Can you work these out from the model? Positions are in its coordinate system, mm. Coordinates: 2 decimals unless noted, no trailing zeros. Order: outer loops, then holes, each group sorted by start corner. A loop starts at its lowest first (then second) coordinate and runs counter-clockwise, first axis right, second up. Notation, with made-up numbers: M -4,-9.75 L 16,-9.75 A22 cw 16,6.25 Z; hole C 86,76.5 d8. An arc over 180 degrees is marked long. Answer as a JSON object with one key per item and string values.
from build123d import *

# Parameters (mm, degrees)
SKETCH1_R           = 2.5
BOSS_EXTRUDE1_DEPTH = 3.175
FILLET1_R           = 10
SKETCH2_W           = 9
SKETCH2_H           = 21
CUT_EXTRUDE1_DEPTH  = 90.108082017
FILLET2_R           = 10
SKETCH4_W           = 90.343709808
SKETCH4_H           = 29.159436912
CUT_EXTRUDE3_DEPTH  = 83
CUT_EXTRUDE4_DEPTH  = 90.108082017


with BuildPart() as part:
    # Sketch1 → Boss-Extrude1 (new body)
    with BuildSketch(Plane.XY):
        with BuildLine():
            Line((-9.56, -38.262636689), (-9.56, -41.437636689))
            Line((-9.56, -41.437636689), (9.56, -41.437636689))
            Line((9.56, -41.437636689), (9.56, -38.262636689))
            Line((9.56, -38.262636689), (12.735, -38.262636689))
            Line((12.735, -38.262636689), (12.735, -41.437636689))
            Line((12.735, -41.437636689), (15.91, -41.437636689))
            Line((15.91, -41.437636689), (21.91, -41.437636689))
            Line((21.91, -41.437636689), (21.91, -32.437636689))
            Line((21.91, -32.437636689), (18.735, -32.437636689))
            Line((18.735, -32.437636689), (18.735, -20.437636689))
            Line((18.735, -20.437636689), (21.91, -20.437636689))
            Line((21.91, -20.437636689), (21.91, -9.437636689))
            Line((21.91, -9.437636689), (40, -9.437636689))
            Line((40, -9.437636689), (40, 30.562363311))
            Line((40, 30.562363311), (10, 30.562363311))
            Line((10, 30.562363311), (10, 45.562363311))
            Line((10, 45.562363311), (10, 48.89577614))
            Line((10, 48.89577614), (22.410269523, 48.89577614))
            ThreePointArc((22.410269523, 48.89577614), (26.000000001, 52.562363311), (22.410269523, 56.228950483))
            Line((22.410269523, 56.228950483), (11.727794547, 56.228950483))
            Line((11.727794547, 56.228950483), (11.727794547, 59.562363311))
            Line((11.727794547, 59.562363311), (10, 59.562363311))
            Line((10, 59.562363311), (8.552794547, 59.562363311))
            Line((8.552794547, 59.562363311), (8.552794547, 62.737363311))
            Line((8.552794547, 62.737363311), (11.727794547, 62.737363311))
            Line((11.727794547, 62.737363311), (11.727794547, 74.562363311))
            Line((11.727794547, 74.562363311), (40, 74.562363311))
            Line((40, 74.562363311), (40, 79.562363311))
            Line((40, 79.562363311), (0, 79.562363311))
            Line((0, 79.562363311), (-40, 79.562363311))
            Line((-40, 79.562363311), (-40, 74.562363311))
            Line((-40, 74.562363311), (-11.727794547, 74.562363311))
            Line((-11.727794547, 74.562363311), (-11.727794547, 62.737363311))
            Line((-11.727794547, 62.737363311), (-8.552794547, 62.737363311))
            Line((-8.552794547, 62.737363311), (-8.552794547, 59.562363311))
            Line((-8.552794547, 59.562363311), (-10, 59.562363311))
            Line((-10, 59.562363311), (-11.727794547, 59.562363311))
            Line((-11.727794547, 59.562363311), (-11.727794547, 56.228950483))
            Line((-11.727794547, 56.228950483), (-22.410269523, 56.228950483))
            ThreePointArc((-22.410269523, 56.228950483), (-26.000000001, 52.562363311), (-22.410269523, 48.89577614))
            Line((-22.410269523, 48.89577614), (-10, 48.89577614))
            Line((-10, 48.89577614), (-10, 45.562363311))
            Line((-10, 45.562363311), (-10, 30.562363311))
            Line((-10, 30.562363311), (-40, 30.562363311))
            Line((-40, 30.562363311), (-40, -9.437636689))
            Line((-40, -9.437636689), (-21.91, -9.437636689))
            Line((-21.91, -9.437636689), (-21.91, -20.437636689))
            Line((-21.91, -20.437636689), (-18.735, -20.437636689))
            Line((-18.735, -20.437636689), (-18.735, -32.437636689))
            Line((-18.735, -32.437636689), (-21.91, -32.437636689))
            Line((-21.91, -32.437636689), (-21.91, -41.437636689))
            Line((-21.91, -41.437636689), (-15.91, -41.437636689))
            Line((-15.91, -41.437636689), (-12.735, -41.437636689))
            Line((-12.735, -41.437636689), (-12.735, -38.262636689))
            Line((-12.735, -38.262636689), (-9.56, -38.262636689))
        make_face()
        with BuildLine():
            Line((4, 1.562363311), (-4, 1.562363311))
            ThreePointArc((-4, 1.562363311), (-4.707106781, 1.85525653), (-5, 2.562363311))
            Line((-5, 2.562363311), (-5, 3.562363311))
            ThreePointArc((-5, 3.562363311), (-4.707106781, 4.269470092), (-4, 4.562363311))
            Line((-4, 4.562363311), (4, 4.562363311))
            ThreePointArc((4, 4.562363311), (4.707106781, 4.269470092), (5, 3.562363311))
            Line((5, 3.562363311), (5, 2.562363311))
            ThreePointArc((5, 2.562363311), (4.707106781, 1.85525653), (4, 1.562363311))
        make_face(mode=Mode.SUBTRACT)
        with Locations((-22, 52.562363311)):
            Circle(SKETCH1_R, mode=Mode.SUBTRACT)
        with Locations((22, 52.562363311)):
            Circle(SKETCH1_R, mode=Mode.SUBTRACT)
    extrude(amount=BOSS_EXTRUDE1_DEPTH)

    # Fillet1
    # the kernel refuses this fillet: 10 mm, written as the material it takes off along each edge
    with BuildSketch(Plane(origin=(-40, 79.562363311, -21.650635095), x_dir=(0, -1, 0), z_dir=(0, 0, 1))) as fillet1_piece_1:
        with BuildLine():
            CenterArc((10, 8.660254038), FILLET1_R, 180, 60)
            Line((0, 8.660254038), (-0.2, 8.660254038))
            Line((-0.2, 8.660254038), (-0.2, 0))
            Line((-0.2, 0), (0, -0.2))
            ThreePointArc((0, -0.2), (2.5, -0.2), (4.9, -0.173205081))
            Line((4.9, -0.173205081), (5, 0))
        make_face()
    extrude(amount=46.476270189, mode=Mode.SUBTRACT)
    with BuildSketch(Plane(origin=(40, 79.562363311, -21.650635095), x_dir=(-1, 0, 0), z_dir=(0, 0, 1))) as fillet1_piece_2:
        with BuildLine():
            CenterArc((8.660254038, 10), FILLET1_R, 210, 60)
            Line((0, 5), (-0.173205081, 4.9))
            ThreePointArc((-0.173205081, 4.9), (-0.2, 2.5), (-0.2, 0))
            Line((-0.2, 0), (0, -0.2))
            Line((0, -0.2), (8.660254038, -0.2))
            Line((8.660254038, -0.2), (8.660254038, 0))
        make_face()
    extrude(amount=46.476270189, mode=Mode.SUBTRACT)

    # Sketch2 → Cut-Extrude1 (cut, through all)
    with BuildSketch(Plane.XY.offset(3.175)):
        with Locations((-12.61, -26.137636689)):
            Rectangle(SKETCH2_W, SKETCH2_H)
    extrude(amount=-CUT_EXTRUDE1_DEPTH, mode=Mode.SUBTRACT)

    # Fillet2
    fillet2_edges = [part.edges().sort_by_distance(p)[0] for p in [
        (40, 30.562363311, 1.5875),
        (40, -9.437636689, 1.5875),
        (-40, -9.437636689, 1.5875),
        (-40, 30.562363311, 1.5875),
    ]]
    fillet(fillet2_edges, radius=FILLET2_R)

    # Sketch4 → Cut-Extrude3 (cut)
    with BuildSketch(Plane.XZ.offset(41.437636689)):
        Rectangle(SKETCH4_W, SKETCH4_H)
    extrude(amount=-CUT_EXTRUDE3_DEPTH, mode=Mode.SUBTRACT)

    # Sketch5 → Cut-Extrude4 (cut, through all)
    with BuildSketch(Plane.XY.offset(3.175)):
        Polygon((6.2, 68.212363311), (-6.2, 68.212363311), (-6.2, 45.562363311), (-3, 45.562363311), (-3, 40.562363311), (-0.113822398, 40.562363311), (0.113822398, 40.562363311), (3, 40.562363311), (3, 45.562363311), (6.2, 45.562363311), align=None)
    extrude(amount=-CUT_EXTRUDE4_DEPTH, mode=Mode.SUBTRACT)


solid = part.part
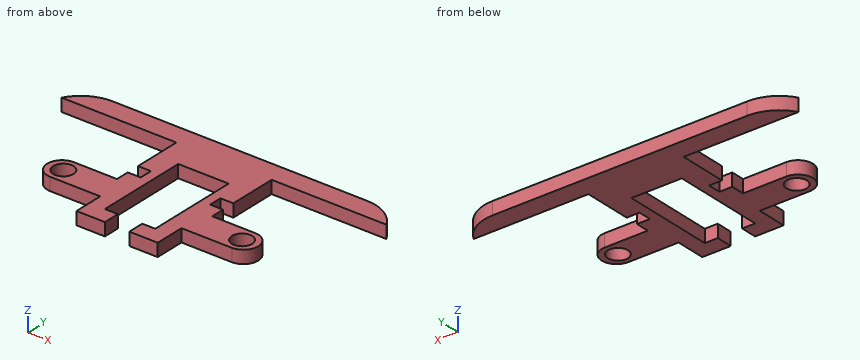
Item 1: I'm going to push flat-ended pins straight in: pin 1 (1 mm diameter, centred on y = 74, z = 0.5, fed in from -X); pin 2 (1 mm diameter, centred on y = 61, z = 1, fed in from -X); pin 3 (1.6 mm diameter, centred on y = 61, z = 1.5, fed in from +X). Where does each tip first touch, or does it pass through?
Answers follow:
{"pin 1": "stops at x = -11.73", "pin 2": "stops at x = -8.55", "pin 3": "stops at x = 8.55"}
Item 2: I want a section at C-C, the plane z = 1.9. Give the number of separate pieces and of enclosed holes in the cut face, plus the area to 3 significant figures.
Answers follow:
{"separate pieces": "1", "enclosed holes": "2", "area": "957 mm^2"}
Item 3: I want a section at B-B, the plane y = 67. Write out the boundary of the cut face in (x, z) (3 decimals).
Answers follow:
{"outline": "M -11.728,0 L -6.2,0 L -6.2,3.175 L -11.728,3.175 Z; M 6.2,0 L 11.728,0 L 11.728,3.175 L 6.2,3.175 Z"}
Item 4: I want a section at A-A, the plane y = 48. Write out the boundary of the cut face in (x, z) (3 decimals).
Answers follow:
{"outline": "M -10,0 L -6.2,0 L -6.2,3.175 L -10,3.175 Z; M 6.2,0 L 10,0 L 10,3.175 L 6.2,3.175 Z"}
Item 5: Please list where these lines run through material, in increasing order: line 1 (Y direction, x = 22, z = 2.15); line 2 (X direction, y = 58.5, z = 1.45); line 3 (Y direction, x = 16, z = 2.25).
Answers follow:
{"line 1": "y = 48.9 to 50.06, 55.06 to 56.23, 74.56 to 79.56", "line 2": "x = -11.73 to -6.2, 6.2 to 11.73", "line 3": "y = 48.9 to 56.23, 74.56 to 79.56"}
Item 6: I want a section at D-D, the plane x = 30. Write out the boundary of the cut face in (y, z) (3 decimals).
Answers follow:
{"outline": "M 74.562,0 L 79.562,0 L 79.562,3.175 L 74.562,3.175 Z"}
